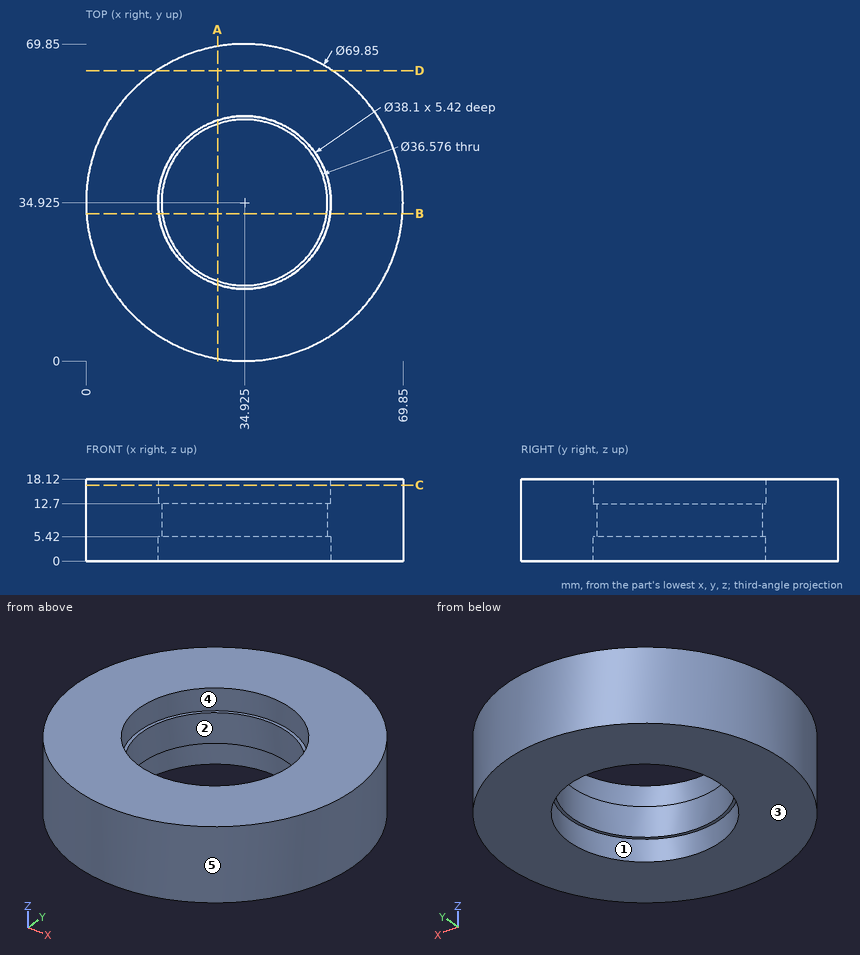
Could you check a few things on this drawing? It's one solid part, dimensions in mm from its lowest x, y, z. A direction names the side the tool comes from. Round coordinates to 2 decimals unless told otherwise and drop trailing zeros. Order: outer loops, then holes, each group sorted by start corner. A loop starts at its lowest first (then second) coordinate and runs counter-clockwise, first axis right, second up.
Q1. Imagine slicing it at A-A, the plane x = 29. List the corners of the cut face in (y, z) for me, then the cut area to 3 significant figures.
Geometry says:
outline: (0.51, 0) - (16.82, 0) - (16.82, 5.42) - (17.62, 5.42) - (17.62, 12.7) - (16.82, 12.7) - (16.82, 18.12) - (0.51, 18.12) - close; (52.23, 5.42) - (53.03, 5.42) - (53.03, 0) - (69.34, 0) - (69.34, 18.12) - (53.03, 18.12) - (53.03, 12.7) - (52.23, 12.7) - close
area: 603 mm2
Q2. Thinking about a two-plate mould opening in X: for the marked faces 3, 4 and 5, which applies, released by +X, released by -X, zero draft, split by the parting line, or undercut?
Geometry says:
face 3: zero draft
face 4: undercut
face 5: split by the parting line
Q3. Which directions (+Z, -Z, +X, -X, +Y, -Y) give clear straight access to the entire face, cutting with the end or side of a thin tool? Please do the marked faces 1 and 2.
Geometry says:
face 1: -Z
face 2: +Z, -Z
Q4. Imagine slicing it at B-B, the plane y = 32.5. List the corners of the cut face in (x, z) for me, then the cut area to 3 significant figures.
Geometry says:
outline: (0.08, 0) - (16.03, 0) - (16.03, 5.42) - (16.8, 5.42) - (16.8, 12.7) - (16.03, 12.7) - (16.03, 18.12) - (0.08, 18.12) - close; (53.05, 5.42) - (53.82, 5.42) - (53.82, 0) - (69.77, 0) - (69.77, 18.12) - (53.82, 18.12) - (53.82, 12.7) - (53.05, 12.7) - close
area: 589 mm2
Q5. Imagine slicing it at D-D, the plane y = 64. List the corners of the cut face in (x, z) for me.
Geometry says:
outline: (15.58, 0) - (54.27, 0) - (54.27, 18.12) - (15.58, 18.12) - close
Q6. Please list where these lines run through material, in increasing order: probe 1 along Y at (x, z) = (35, 3.75); probe 2 along Y at (x, z) = (34.5, 12.5); probe 3 along X at (y, z) = (19.5, 10.5).
Geometry says:
probe 1: y = 0 to 15.88, 53.97 to 69.85
probe 2: y = 0 to 16.64, 53.21 to 69.85
probe 3: x = 3.59 to 25.1, 44.75 to 66.26
Q7. Imagine slicing it at C-C, the plane z = 16.75. List the corners of the cut face in (x, y) for me (3 decimals), then the cut area to 3 significant figures.
Geometry says:
outline: circle Ø69.85 at (34.925, 34.925); hole circle Ø38.1 at (34.925, 34.925)
area: 2,690 mm2
Q8. I'm going to push flat-ended pins straight in: P1, Ø1.5, axis at x = 48, z = 15.5, coming from the -Y side; P2, Ø3, axis at y = 44.5, z = 5.5, coming from the +X side; P3, Ø1.5, axis at x = 49, z = 13, coming from the +Y side. Where does each tip first touch, or does it pass through?
Geometry says:
P1: stops at y = 2.25
P2: stops at x = 68.9
P3: stops at y = 67.21
